```python
from build123d import *

# Parameters (mm, degrees)
EXTRUDE_1_DEPTH     = 2
CUT_EXTRUDE_2_DEPTH = 59.758033272
SKETCH_3_R          = 1.5
CUT_EXTRUDE_1_DEPTH = 59.758033272


with BuildPart() as part:
    # 草图1 → 凸台-拉伸1 (new body)
    with BuildSketch(Plane.XY):
        with BuildLine():
            Line((-35.244286067, 2.232984072), (14.755713933, 2.232984072))
            ThreePointArc((14.755713933, 2.232984072), (22.255713134, -5.267016727), (14.755712334, -12.767015928))
            Line((14.755712334, -12.767015928), (-2.744287666, -12.767015928))
            Line((-2.744287666, -12.767015928), (-2.744287666, -32.767015928))
            ThreePointArc((-2.744287666, -32.767015928), (-10.244286561, -40.267014822), (-17.744285455, -32.767015928))
            Line((-17.744285455, -32.767015928), (-17.744285455, -12.767015928))
            Line((-17.744285455, -12.767015928), (-35.244285455, -12.767015928))
            ThreePointArc((-35.244285455, -12.767015928), (-42.744286067, -5.267016233), (-35.244286067, 2.232984072))
        make_face()
    extrude(amount=EXTRUDE_1_DEPTH)

    # 草图2 → 切除-拉伸2 (cut, through all)
    with BuildSketch(Plane.XY.offset(2)):
        with BuildLine():
            Line((-11.744285455, -3.767015928), (-11.744285455, -30.635435278))
            ThreePointArc((-11.744285455, -30.635435278), (-10.244286561, -32.135434173), (-8.744287666, -30.635435278))
            Line((-8.744287666, -30.635435278), (-8.744287666, -3.767015928))
            ThreePointArc((-8.744287666, -3.767015928), (-10.244286561, -2.267017033), (-11.744285455, -3.767015928))
        make_face()
    extrude(amount=-CUT_EXTRUDE_2_DEPTH, mode=Mode.SUBTRACT)

    # 草图3 → 切除-拉伸1 (cut, through all)
    with BuildSketch(Plane(origin=(0, 0, 0), x_dir=(-1, 0, 0), z_dir=(0, 0, -1))):
        with Locations((-14.755712334, -5.267015928)):
            Circle(SKETCH_3_R)
        with Locations((35.244285455, -5.267015928)):
            Circle(SKETCH_3_R)
    extrude(amount=-CUT_EXTRUDE_1_DEPTH, mode=Mode.SUBTRACT)


solid = part.part
```
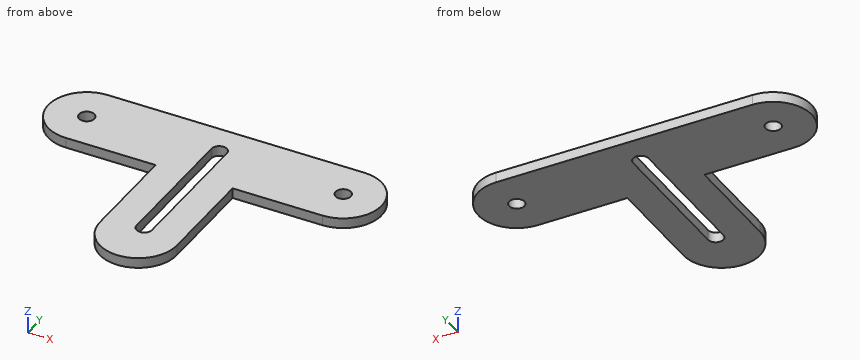
Here's how the part is built. I have some questions about the finished solid (model axes, mm). Give positions to 0.01 mm unless a question says otherwise; leave off trailing zeros. Order: outer loops, then holes, each group sorted by start corner. A loop starts at its lowest first (then second) coordinate and runs counter-clockwise, first axis right, second up. Notation, with made-up numbers: (31, -8.5) - (90, -8.5) arc R27 cw to (90, 18.5) - close; hole circle Ø6 at (25.25, 37.5). An arc over 180 degrees is marked (long way). Answer as a JSON object with one key per item and string values. Group by question number.
Item 1: If we section it at C-C on y = -3: Please give me the cut outline in (x, z), and give its area (3 significant figures).
Item 2: Please list where these lines run through material, in increasing order: probe 1 along X at (y, z) = (-30, 0.1); probe 2 along Y at (x, z) = (-19.5, 1.5); probe 3 along Y at (x, z) = (15.5, 1.05).
Item 3: If we section it at B-B on z = 1.05: Please give me the cut outline in (x, y).
Item 4: If we section it at D-D on x = -25: Please give me the cut outline in (y, z), and give its area (3 significant figures).
Item 5: For P1, Ø1, axis at x = 9.5, z = 1, coming from the -Y side; P2, Ø2.5, axis at x = -35.24, y = -5.27, coming from the +Z side; P3, Ø0.6, axis at y = -22, z = 1, coming from the -X side; P4, Ø1, axis at y = -21.5, z = 0.5, coming from the +X side, each with a flat end and sliding along its axis, tell me the tip position at first contact or that it passes through.
Item 6: If we section it at A-A on y = -30: Please give me the cut outline in (x, z), and give its area (3 significant figures).
Result set:
{
 "1": {"outline": "(-42.39, 0) - (-11.53, 0) - (-11.53, 2) - (-42.39, 2) - close; (-8.96, 0) - (21.9, 0) - (21.9, 2) - (-8.96, 2) - close", "area": "123 mm²"},
 "2": {"probe 1": "-17.74 to -11.74, -8.74 to -2.74", "probe 2": "-12.77 to 2.23", "probe 3": "-12.73 to -6.57, -3.96 to 2.2"},
 "3": {"outline": "(-35.24, -12.77) - (-17.74, -12.77) - (-17.74, -32.77) arc R7.5 ccw to (-2.74, -32.77) - (-2.74, -12.77) - (14.76, -12.77) arc R7.5 ccw to (14.76, 2.23) - (-35.24, 2.23) arc R7.5 ccw to start; hole circle Ø3 at (-35.24, -5.27); hole (-11.74, -30.64) arc R1.5 ccw to (-8.74, -30.64) - (-8.74, -3.77) arc R1.5 ccw to (-11.74, -3.77) - close; hole circle Ø3 at (14.76, -5.27)"},
 "4": {"outline": "(-12.77, 0) - (2.23, 0) - (2.23, 2) - (-12.77, 2) - close", "area": "30.0 mm²"},
 "5": {"P1": "y = -12.77", "P2": "through", "P3": "x = -17.74", "P4": "x = -2.74"},
 "6": {"outline": "(-17.74, 0) - (-11.74, 0) - (-11.74, 2) - (-17.74, 2) - close; (-8.74, 0) - (-2.74, 0) - (-2.74, 2) - (-8.74, 2) - close", "area": "24.0 mm²"}
}
